Input: part model. Units: mm. Frame: model coordinates. Face numbers are marked on the shaded views. A direction names the side the tool comes from. Give positions to 0.01 mm unless a question says otherwise; leave off trailing zeros. Loops run counter-clockwise (first coordinate to the right, second up) from the corner with the lowest first, then second, coordinate; pieces in that order, holes last. Notation, with made-up numbers: M 27.25,60.5 L 31.25,60.5 A14 cw 31.25,87.5 Z; hole C -31.5,38 d6. An arc over 180 degrees is marked long. Answer as a JSON object with one key per item and string values. Group by question number.
1) Section query C-C on z = 0. Return loops of the section in (x, y).
2) Access query for the marked faces 1, 2 and 3. Directions: +Z, -Z, +X, -X, +Y, -Y. A direction counts if a zero-diameter tool reaches every point of the face in a straight line with its end or side. Return the directions, or none.
3) Ray query, L1, parallel to X at y = 16, z = -21; L2, parallel to Y at x = -17, z = -17; L3, parallel to Z at x = 10, y = 32. Return the intervals inside material, ascending.
4) Section query B-B on y = 6. Return loops of the section in (x, z).
5) First-contact query: P1, Ø4, axis at x = -17.5, y = 11, coming from the -Z side; P2, Ø4, axis at x = -17, y = 7, coming from the +Z side; P3, Ø4, axis at x = -2.5, y = 28, coming from the +Z side. Flat tips, straight axial feed; report the tip coordinate or a pass-through.
6) Section query D-D on x = 8. Return loops of the section in (y, z).
7) Section query A-A on x = 0. Return loops of the section in (y, z), plus the area to 3 significant figures.
8) Draft query along X for the marked faces 4, 5, 6 and 7. Return one class per face: +X half, -X half, draft (parallel to the pull), parting line (faces both ways), or undercut.
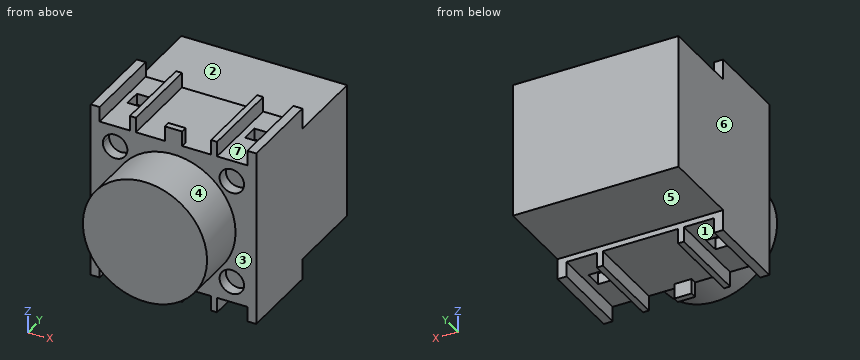
from build123d import *

# Parameters (mm, degrees)
F0_R      = 3.25
F0_R_2    = 16.5
F1_DEPTH  = 22.2
F2_W      = 4.6
F2_H      = 20.5
F3_DEPTH  = 4
F4_W      = 4.6
F4_H      = 20.5
F5_DEPTH  = 4
F6_DEPTH  = 3
F7_DEPTH  = 13.7
F8_W      = 44
F8_H      = 36
F9_DEPTH  = 21.5
F10_W     = 4.527392
F10_H     = 4.484308
F12_DEPTH = 3
F11_W     = 4.516719
F11_H     = 4.586656
F11_W_2   = 4.516715
F11_H_2   = 4.484454
F13_DEPTH = 3


with BuildPart() as f1:
    # F0 (on Front) → F1 (new body)
    with BuildSketch(Plane.XZ):
        Polygon((19.62, -23.5), (22, -23.5), (22, -19.5), (22, 19.5), (22, 23.5), (19.62, 23.5), (19.62, 19.5), (11.58, 19.5), (11.58, 23.5), (9.98, 23.5), (9.98, 19.5), (2.3, 19.5), (2.3, 23.5), (-2.3, 23.5), (-2.3, 19.5), (-9.98, 19.5), (-9.98, 23.5), (-11.58, 23.5), (-11.58, 19.5), (-19.62, 19.5), (-19.62, 23.5), (-22, 23.5), (-22, 19.5), (-22, 13.9), (-22, -19.5), (-22, -23.5), (-19.62, -23.5), (-19.62, -19.5), (-11.58, -19.5), (-11.58, -23.5), (-9.98, -23.5), (-9.98, -19.5), (-2.3, -19.5), (-2.3, -23.5), (2.3, -23.5), (2.3, -19.5), (9.98, -19.5), (9.98, -23.5), (11.58, -23.5), (11.58, -19.5), (19.62, -19.5), align=None)
        with Locations((-15.500009, -13.888962)):
            Circle(F0_R, mode=Mode.SUBTRACT)
        with Locations((15.500009, -13.888962)):
            Circle(F0_R, mode=Mode.SUBTRACT)
        with BuildLine():
            ThreePointArc((-12.250009, 13.888962), (-15.502769, 10.638963), (-18.750005, 13.894481))
            ThreePointArc((-18.750005, 13.894481), (-15.49725, 17.13896), (-12.250009, 13.888962))
        make_face(mode=Mode.SUBTRACT)
        Circle(F0_R_2, mode=Mode.SUBTRACT)
        with Locations((15.500009, 13.888962)):
            Circle(F0_R, mode=Mode.SUBTRACT)
        with BuildLine():
            ThreePointArc((-12.250009, 13.888962), (-15.49725, 17.13896), (-18.750005, 13.894481))
            ThreePointArc((-18.750005, 13.894481), (-15.502769, 10.638963), (-12.250009, 13.888962))
        make_face()
        with Locations((15.500009, 13.888962)):
            Circle(F0_R)
        Circle(F0_R_2)
        with Locations((-15.500009, -13.888962)):
            Circle(F0_R)
        with Locations((15.500009, -13.888962)):
            Circle(F0_R)
    extrude(amount=-F1_DEPTH)

    # F2 (on face) → F3 (cut)
    with BuildSketch(Plane.XY.offset(23.5)):
        with Locations((0, 11.95)):
            Rectangle(F2_W, F2_H)
    extrude(amount=-F3_DEPTH, mode=Mode.SUBTRACT)

    # F4 (on face) → F5 (cut)
    with BuildSketch(Plane(origin=(0, 0, -23.5), x_dir=(1, 0, 0), z_dir=(0, 0, -1))):
        with Locations((0, -11.95)):
            Rectangle(F4_W, F4_H)
    extrude(amount=-F5_DEPTH, mode=Mode.SUBTRACT)

    # F0 (on Front) → F6 (cut)
    with BuildSketch(Plane.XZ):
        with BuildLine():
            ThreePointArc((-12.250009, 13.888962), (-15.49725, 17.13896), (-18.750005, 13.894481))
            ThreePointArc((-18.750005, 13.894481), (-15.502769, 10.638963), (-12.250009, 13.888962))
        make_face()
        with Locations((15.500009, 13.888962)):
            Circle(F0_R)
        with Locations((15.500009, -13.888962)):
            Circle(F0_R)
        with Locations((-15.500009, -13.888962)):
            Circle(F0_R)
    extrude(amount=-F6_DEPTH, mode=Mode.SUBTRACT)

    # F0 (on Front) → F7 (join)
    with BuildSketch(Plane.XZ):
        Circle(F0_R_2)
    extrude(amount=F7_DEPTH)

    # F8 (on face) → F9 (join)
    with BuildSketch(Plane(origin=(0, 22.2, 0), x_dir=(-1, 0, 0), z_dir=(0, 1, 0))):
        Rectangle(F8_W, F8_H)
    extrude(amount=F9_DEPTH)

    # F10 (on face) → F12 (cut)
    with BuildSketch(Plane.XY.offset(19.5)):
        with Locations((-15.6, 12.5)):
            Rectangle(F10_W, F10_H)
        Polygon((13.336304, 10.257846), (15.6, 10.257846), (17.863696, 10.257846), (17.863696, 14.742154), (13.336304, 14.742154), align=None)
    extrude(amount=-F12_DEPTH, mode=Mode.SUBTRACT)

    # F11 (on face) → F13 (cut)
    with BuildSketch(Plane(origin=(0, 0, -19.5), x_dir=(1, 0, 0), z_dir=(0, 0, -1))):
        with Locations((15.625707, -12.502325)):
            Rectangle(F11_W, F11_H)
        with Locations((-15.580125, -12.502325)):
            Rectangle(F11_W_2, F11_H_2)
    extrude(amount=-F13_DEPTH, mode=Mode.SUBTRACT)


solid = f1.part
Output:
{
 "1": {"outline": "M -22,0 L -16.5,0 L -16.5,-13.7 L 16.5,-13.7 L 16.5,0 L 22,0 L 22,43.7 L -22,43.7 Z"},
 "2": {"face 1": "-Z, +Y, -Y", "face 2": "+Z, +X, -X, +Y", "face 3": "-Y"},
 "3": {"L1": "x = -22 to -19.62, -11.58 to -9.98, 9.98 to 11.58, 19.62 to 22", "L2": "y = 0 to 10.26, 14.74 to 43.7", "L3": "z = -18 to 18"},
 "4": {"outline": "M -22,-23.5 L -19.62,-23.5 L -19.62,-19.5 L -11.58,-19.5 L -11.58,-23.5 L -9.98,-23.5 L -9.98,-19.5 L 9.98,-19.5 L 9.98,-23.5 L 11.58,-23.5 L 11.58,-19.5 L 19.62,-19.5 L 19.62,-23.5 L 22,-23.5 L 22,23.5 L 19.62,23.5 L 19.62,19.5 L 11.58,19.5 L 11.58,23.5 L 9.98,23.5 L 9.98,19.5 L -9.98,19.5 L -9.98,23.5 L -11.58,23.5 L -11.58,19.5 L -19.62,19.5 L -19.62,23.5 L -22,23.5 Z"},
 "5": {"P1": "stops at z = -19.5", "P2": "stops at z = 19.5", "P3": "stops at z = 18"},
 "6": {"outline": "M -13.7,-14.43 L 0,-14.43 L 0,-19.5 L 22.2,-19.5 L 22.2,-18 L 43.7,-18 L 43.7,18 L 22.2,18 L 22.2,19.5 L 0,19.5 L 0,14.43 L -13.7,14.43 Z"},
 "7": {"outline": "M -13.7,-16.5 L 0,-16.5 L 0,-23.5 L 1.7,-23.5 L 1.7,-19.5 L 22.2,-19.5 L 22.2,-18 L 43.7,-18 L 43.7,18 L 22.2,18 L 22.2,19.5 L 1.7,19.5 L 1.7,23.5 L 0,23.5 L 0,16.5 L -13.7,16.5 Z", "area": "2,110 mm^2"},
 "8": {"face 4": "parting line", "face 5": "draft", "face 6": "-X half", "face 7": "undercut"}
}
